Input: part model. Units: mm. Frame: model coordinates. Face numbers are marked on the shaded views. A direction names the side the tool comes from. Give positions to 0.01 mm unless a question says otherwise; leave off trailing zeros. Loops run counter-clockwise (first coordinate to the right, second up) from the corner with the lowest first, then second, coordinate; pieces in that order, holes last. Notation, with made-up numbers: (73, -18) -> (77, -18) arc R18 cw to (77, -2) -> close; hole circle Ø10 at (-6, 73.5). An arc over 180 degrees is marked (long way). Answer in a Markdown table with one row per item. Add a question column.
```python
from build123d import *

# Parameters (mm, degrees)
CHAMFER1_SIZE      = 0.2
CHAMFER1_SIZE2     = 0.346410162
CUT_EXTRUDE1_DEPTH = 0.8
CUT_EXTRUDE1_TAPER = 6


with BuildPart() as part:
    # Sketch1 → Revolve1 (revolve)
    with BuildSketch(Plane.XY, mode=Mode.PRIVATE) as revolve1_sk:
        with BuildLine():
            Line((-1.6, 0), (8.4, 0))
            Line((8.4, 0), (8.4, 1.1))
            Line((8.4, 1.1), (0, 1.1))
            Line((0, 1.1), (-0.869043005, 1.969043005))
            ThreePointArc((-0.869043005, 1.969043005), (-0.992640239, 2.010371092), (-1.1, 1.936491673))
            ThreePointArc((-1.1, 1.936491673), (-1.472983346, 1), (-1.6, 0))
        make_face()
    revolve(revolve1_sk.sketch.rotate(Axis((0, 0, 0), (1, 0, 0)), 90), axis=Axis((0, 0, 0), (1, 0, 0)))

    # Chamfer1
    chamfer1_edges = [part.edges().sort_by_distance(p)[0] for p in [
        (8.4, 0, -1.1),
    ]]
    chamfer1_side = [part.faces().sort_by_distance(p)[0] for p in [
        (8.4, 0, 0),
    ]]
    chamfer(chamfer1_edges, length=CHAMFER1_SIZE, length2=CHAMFER1_SIZE2, reference=chamfer1_side[0])

    # Sketch3 → Cut-Extrude1 (cut)
    with BuildSketch(Plane(origin=(-1.6, 0, 0), x_dir=(0, 0, -1), z_dir=(1, 0, 0))):
        Polygon((-0.22, 1.1), (-0.146666667, 0.733333333), (-0.36140157, 0.36140157), (-0.733333333, 0.146666667), (-1.1, 0.22), (-1.1, -0.22), (-0.733333333, -0.146666667), (-0.36140157, -0.36140157), (-0.146666667, -0.733333333), (-0.22, -1.1), (0.22, -1.1), (0.146666667, -0.733333333), (0.36140157, -0.36140157), (0.733333333, -0.146666667), (1.1, -0.22), (1.1, 0.22), (0.733333333, 0.146666667), (0.36140157, 0.36140157), (0.146666667, 0.733333333), (0.22, 1.1), align=None)
    extrude(amount=CUT_EXTRUDE1_DEPTH, taper=CUT_EXTRUDE1_TAPER, mode=Mode.SUBTRACT)


solid = part.part
```
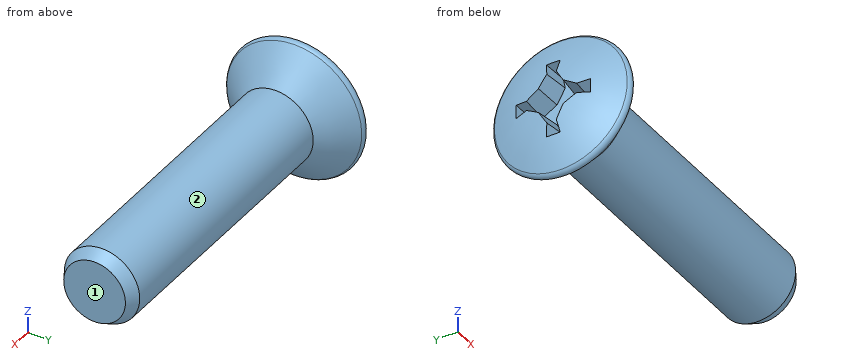
1) Reachability of the marked faces 1 and 2 from +Z, -Z, +X, -X, +Y, -Y: full face, straight path, thin tool, end or side. Return the list, or none.
2) Section A-A on x = 4.25. Output: boundary loops of the cut face in (y, z), and give its area (3 significant figures).
3) Pin query (flat end, axial travel): pin 1 (0.6 mm diameter, centred on y = 0.5, z = 0, fed in from -X); pin 2 (1.5 mm diameter, centred on x = 3.5, y = 1.5, fed in from +Z). Return the tip coordinate at first contact, or that it passes through.
4) Material intervals for line 1 along X through (y, z) = (-0.55, -0.1); line 2 along X through (y, z) = (-0.4, -0.7); line 3 along Y through (x, z) = (7.5, 0.1), sorted ascending.
Working result:
| question | item | result |
|---|---|---|
| 1 | face 1 | +Z, -Z, +X, +Y, -Y |
| 1 | face 2 | +X |
| 2 | outline | circle Ø2.2 at (0, 0) |
| 2 | area | 3.80 mm2 |
| 3 | pin 1 | stops at x = -1.56 |
| 3 | pin 2 | stops at z = 0.8 |
| 4 | line 1 | x = -0.8 to 8.4 |
| 4 | line 2 | x = -1.52 to 8.4 |
| 4 | line 3 | y = -1.1 to 1.1 |
